Geometry check sheet. Reference: the model listing, model coordinates, mm. A direction names the side the tool comes from. Give positions to 0.01 mm unless a question says otherwise; leave off trailing zeros. Write each loop counter-clockwise with the first axis right and the second up, starting at its lowest first coordinate (ties: lowest second). Pieces come first, ordered by that corner, then holes. Notation, with made-up numbers: M -32.5,83.5 L -23.5,83.5 A33 ccw -23.5,115.5 Z; hole C 44,43 d8. An arc over 180 degrees is marked long. One line per item, written item: value. Start each with the question number.
1. Scan lines: line 1 (Y direction, x = 125, z = -196.75); line 2 (Z direction, x = -46, y = 36); line 3 (X direction, y = 16, z = 194). Record each from-to range of solid material in increasing order.
2. Cross-section at A-A on z = 36. Record the cut outline in (x, y), then the cut area to 3 significant figures.
3. Cross-section at B-B on x = -84. Record the cut outline in (y, z), then the cut area to 3 significant figures.
4. Gauge pin test, flat ends, axial feed: pin 1 (7 mm diameter, centred on x = -25, y = 16, fed in from +Z); pin 2 (8 mm diameter, centred on y = 25.5, z = 158, fed in from -X); pin 3 (8 mm diameter, centred on y = 55, z = -100.5, fed in from -X); pin 4 (3 mm diameter, centred on x = 252.5, z = -151, fed in from -Y). Record the tip position at first contact, or that the pin passes through.
5. Release check for a two-part mould opening along Y. For faces 5 (the face through (-208.748, 40, -175)), 6 (the face through (-257.003, 43, 174)), 7 (the face through (82, 40, -4)) record: pulls with the +Y half, pulls with the -Y half, needs draft (parallel to the pull), parting line crosses it, or undercut.
6. Tool access check on faces 1 (the face through (268.435, 53, 172)), 2 (the face through (301, 40, 189.418)), 3 (the face through (300, 15, -172)), 4 (the face through (-219, 15, -174)). Record the directions out of +Z, -Z, +X, -X, +Y, -Y that give a thin tool (end or side, any length) a straight path to the whole face; none if there is none.
from build123d import *

# Parameters (mm, degrees)
BOSS_EXTRUDE1_DEPTH     = 200
CUT_EXTRUDE1_DEPTH      = 1875
CUT_EXTRUDE2_DEPTH      = 1
CUT_EXTRUDE2_DEPTH_BACK = 401
SKETCH9_R               = 4.5
CUT_EXTRUDE8_DEPTH      = 535
SKETCH10_W              = 407.608738225
SKETCH10_H              = 383.631753623
CUT_EXTRUDE9_DEPTH      = 40
SKETCH11_W              = 54.119479529
SKETCH11_H              = 34.252835145
SKETCH11_W_2            = 48.255495223
SKETCH11_H_2            = 39.048232065
CUT_EXTRUDE10_DEPTH     = 25


with BuildPart() as part:
    # Sketch1 → Boss-Extrude1 (new body, symmetric)
    with BuildSketch(Plane.XY):
        Polygon((295, 0), (340, 41.963178876), (340, 78), (-295, 78), (-295, 0), align=None)
    extrude(amount=BOSS_EXTRUDE1_DEPTH, both=True)

    # Sketch2 → Cut-Extrude1 (cut)
    with BuildSketch(Plane.XY.offset(200)):
        Polygon((-247.386799314, 6.256797028), (-295, 63), (-295, 0), (-128, 0), align=None)
    extrude(amount=-CUT_EXTRUDE1_DEPTH, mode=Mode.SUBTRACT)

    # Sketch3 → Cut-Extrude2 (cut, two sides)
    with BuildSketch(Plane.XY.offset(200)) as cut_extrude2_sk:
        Polygon((250.288603953, -1126.47745776), (-206.5, 4.114010674), (-208.74763956, 9.677113801), (-262.275114384, 24), (-1440.216479918, 339.193649301), (-3037.790452197, -1503.448201922), (-1347.285368327, -2969.119308982), align=None)
    extrude(amount=CUT_EXTRUDE2_DEPTH, mode=Mode.SUBTRACT)
    extrude(cut_extrude2_sk.sketch, amount=-CUT_EXTRUDE2_DEPTH_BACK, mode=Mode.SUBTRACT)

    # Sketch9 → Cut-Extrude8 (cut, symmetric)
    with BuildSketch(Plane.XY):
        with Locations((-175, 16)):
            Circle(SKETCH9_R)
        with Locations((-100, 16)):
            Circle(SKETCH9_R)
        with Locations((-25, 16)):
            Circle(SKETCH9_R)
        with Locations((50, 16)):
            Circle(SKETCH9_R)
        with Locations((125, 16)):
            Circle(SKETCH9_R)
        with Locations((-241, 51)):
            Circle(SKETCH9_R)
        with Locations((284.7, 51)):
            Circle(SKETCH9_R)
        with BuildLine():
            Line((-161, 55.5), (189, 55.5))
            ThreePointArc((189, 55.5), (193.5, 51), (189, 46.5))
            Line((189, 46.5), (-161, 46.5))
            ThreePointArc((-161, 46.5), (-165.5, 51), (-161, 55.5))
        make_face()
    extrude(amount=CUT_EXTRUDE8_DEPTH, both=True, mode=Mode.SUBTRACT)

    # Sketch10 → Cut-Extrude9 (cut)
    with BuildSketch(Plane(origin=(0, 0, 0), x_dir=(1, 0, 0), z_dir=(0, 1, 0))):
        with Locations((84.497631613, 1.027585054)):
            Rectangle(SKETCH10_W, SKETCH10_H)
    extrude(amount=CUT_EXTRUDE9_DEPTH, mode=Mode.SUBTRACT)

    # Sketch11 → Cut-Extrude10 (cut, symmetric)
    with BuildSketch(Plane.XZ.offset(-40)):
        with Locations((295.495096106, -172.29176078)):
            Rectangle(SKETCH11_W, SKETCH11_H)
        with Locations((-232.875387171, -174.68945924)):
            Rectangle(SKETCH11_W_2, SKETCH11_H_2)
        with Locations((295.495096106, 172.29176078)):
            Rectangle(SKETCH11_W, SKETCH11_H)
        with Locations((-232.875387171, 174.68945924)):
            Rectangle(SKETCH11_W_2, SKETCH11_H_2)
    extrude(amount=CUT_EXTRUDE10_DEPTH, both=True, mode=Mode.SUBTRACT)


solid = part.part
Report:
1. line 1: y = 0 to 11.5, 20.5 to 46.5, 55.5 to 78
1. line 2: z = -200 to -192.84, 190.79 to 200
1. line 3: x = -208.75 to -179.5, -170.5 to -104.5, -95.5 to -29.5, -20.5 to 45.5, 54.5 to 120.5, 129.5 to 312.16
2. outline: M -295,63 L -262.28,24 L -208.75,9.68 L -206.5,4.11 L -128,0 L -119.31,0 L -119.31,40 L 288.3,40 L 288.3,0 L 295,0 L 340,41.96 L 340,78 L -295,78 Z; hole C -241,51 d9; hole C -175,16 d9; hole M -161,46.5 L 189,46.5 A4.5 ccw 189,55.5 L -161,55.5 A4.5 ccw Z; hole C 284.7,51 d9
2. area: 26,400 mm^2
3. outline: M 0,-200 L 46.5,-200 L 46.5,200 L 0,200 L 0,190.79 L 40,190.79 L 40,-192.84 L 0,-192.84 Z; M 55.5,-200 L 78,-200 L 78,200 L 55.5,200 Z
3. area: 12,300 mm^2
4. pin 1: passes through
4. pin 2: stops at x = -266.89
4. pin 3: stops at x = -291.64
4. pin 4: stops at y = 40
5. face 5: undercut
5. face 6: needs draft
5. face 7: pulls with the -Y half
6. face 1: -Y
6. face 2: none
6. face 3: +X
6. face 4: -X
